```python
from build123d import *

# Parameters (mm, degrees)
CUT_EXTRUDE1_DEPTH      = 25.909837414
CUT_EXTRUDE1_DEPTH_BACK = 25.909837414
SKETCH2_R               = 0.9
CUT_EXTRUDE2_DEPTH      = 25.909837579


with BuildPart() as part:
    # Sketch1 → Revolve1 (revolve)
    with BuildSketch(Plane.XY, mode=Mode.PRIVATE) as revolve1_sk:
        with BuildLine():
            Line((20, 10.5), (-10.5, 10.5))
            ThreePointArc((-10.5, 10.5), (-8.266728857, 10.259751459), (-6.135655834, 9.55))
            Line((-6.135655834, 9.55), (20, 9.55))
            Line((20, 9.55), (20, 10.5))
        make_face()
    revolve(revolve1_sk.sketch.rotate(Axis((0, 0, 0), (1, 0, 0)), 90), axis=Axis((0, 0, 0), (1, 0, 0)))

    # Sketch1_3 → Cut-Extrude1 (cut, two sides: drawn at the far end of the back side and taken through both)
    with BuildSketch(Plane.XY.offset(-CUT_EXTRUDE1_DEPTH_BACK)):
        with BuildLine():
            ThreePointArc((-10.5, -10.5), (-0.240248541, -2.233271143), (-6.135655834, 9.55))
            Line((-6.135655834, 9.55), (-10.5, 9.55))
            Line((-10.5, 9.55), (-10.5, -10.5))
        make_face()
        with BuildLine():
            Line((-10.5, 9.55), (-6.135655834, 9.55))
            ThreePointArc((-6.135655834, 9.55), (-8.266728857, 10.259751459), (-10.5, 10.5))
            Line((-10.5, 10.5), (-10.5, 9.55))
        make_face()
        with BuildLine():
            Line((-10.5, 9.55), (-6.135655834, 9.55))
            ThreePointArc((-6.135655834, 9.55), (-8.266728857, 10.259751459), (-10.5, 10.5))
            Line((-10.5, 10.5), (-10.5, 9.55))
        make_face()
    extrude(amount=CUT_EXTRUDE1_DEPTH + CUT_EXTRUDE1_DEPTH_BACK, mode=Mode.SUBTRACT)

    # Sketch2 → Cut-Extrude2 (cut, through all)
    with BuildSketch(Plane.XY):
        with Locations((2, 0)):
            Circle(SKETCH2_R)
    extrude(amount=-CUT_EXTRUDE2_DEPTH, mode=Mode.SUBTRACT)


solid = part.part
```
Build history of the part. All positions in model axes, mm. Coordinates: 2 decimals unless noted, no trailing zeros. Order: outer loops, then holes, each group sorted by start corner. A loop starts at its lowest first (then second) coordinate and runs counter-clockwise, first axis right, second up. Notation, with made-up numbers: (-11.5, 1) -> (-5.5, 1) arc R18 cw to (-5.5, 32) -> close; hole circle Ø4 at (62, 10.25). An arc over 180 degrees is marked (long way). Answer in a Markdown table with one row per item. Add a question column.
Q1. Band-saw the part on B-B, the plane z = -1. List the corners of the cut face in (x, y), then the cut area to 3 significant figures.
Q2. Band-saw the part on D-D, the plane y = -6. List the corners of the cut face in (x, z), then the cut area to 3 significant figures.
Q3. Drop flat-ended pins along their axis: pin 1 (10 mm diameter, centred on x = 9.5, z = -7.5, fed in from -Y); pin 2 (4 mm diameter, centred on x = 1.5, y = -6, fed in from +Z); pin 3 (5 mm diameter, centred on x = 11, y = 5, fed in from -Z). Give the stop position or say it passes through.
Q4. Mould opens along X. For faces 1 (the face through (2.86, 0.27, -10)), 2 (the face through (20, 9, -5)) say: +X half, -X half, draft (parallel to the pull), parting line (faces both ways), or undercut.
Q5. Band-saw the part on C-C, the plane x = -1.5. List the corners of the cut face in (y, z), then the cut area to 3 significant figures.
Q6. Wall check: line 1 along X through (y, z) = (0, -9.75); line 2 along Y through (x, z) = (12.5, 0); line 3 along Z through (x, y) = (18.5, 2.5). Give the ranges that are in metal, low to high. Write a range as [from, to].
Q7. Band-saw the part on A-A, the plane y = 0. List the corners of the cut face in (x, z).
Answers follow:
| question | item | result |
|---|---|---|
| 1 | outline | (-9.5, -10.45) -> (20, -10.45) -> (20, -9.5) -> (-6.02, -9.5) arc R10.5 cw to start; (-9.5, 10.45) arc R10.5 cw to (-6.02, 9.5) -> (20, 9.5) -> (20, 10.45) -> close |
| 1 | area | 52.3 mm^2 |
| 2 | outline | (-1.88, -8.62) -> (20, -8.62) -> (20, -7.43) -> (-1.88, -7.43) -> close; (-1.88, 7.43) -> (20, 7.43) -> (20, 8.62) -> (-1.88, 8.62) -> close |
| 2 | area | 52.0 mm^2 |
| 3 | pin 1 | y = -10.2 |
| 3 | pin 2 | z = 9.71 |
| 3 | pin 3 | z = -10.2 |
| 4 | face 1 | undercut |
| 4 | face 2 | +X half |
| 5 | outline | (-5.41, -9) -> (-5.41, -7.87) arc R9.55 cw to (-5.41, 7.87) -> (-5.41, 9) arc R10.5 ccw to start; (5.41, -9) arc R10.5 ccw to (5.41, 9) -> (5.41, 7.87) arc R9.55 cw to (5.41, -7.87) -> close |
| 5 | area | 38.1 mm^2 |
| 6 | line 1 | [0, 1.1], [2.9, 20] |
| 6 | line 2 | [-10.5, -9.55], [9.55, 10.5] |
| 6 | line 3 | [-10.2, -9.22], [9.22, 10.2] |
| 7 | outline | (0, -10.5) -> (1.1, -10.5) -> (1.1, -9.55) -> (0, -9.55) -> close; (0, 9.55) -> (20, 9.55) -> (20, 10.5) -> (0, 10.5) -> close; (2.9, -10.5) -> (20, -10.5) -> (20, -9.55) -> (2.9, -9.55) -> close |
